Design review of the part built by this model. Coordinates are the model's own, in mm. A direction names the side the tool comes from. Round coordinates to 2 decimals unless told otherwise and drop trailing zeros. Order: outer loops, then holes, each group sorted by start corner. A loop starts at its lowest first (then second) coordinate and runs counter-clockwise, first axis right, second up.
from build123d import *

# Parameters (mm, degrees)
SKETCH3_R           = 4
BOSS_EXTRUDE1_DEPTH = 5.5


with BuildPart() as part:
    # Sketch3 → Boss-Extrude1 (new body)
    with BuildSketch(Plane.XY):
        with BuildLine():
            Line((35.572698846, 9), (-28.927301154, 9))
            Line((-28.927301154, 9), (-32.927301154, 1))
            Line((-32.927301154, 1), (-12.087578676, 2.254578437))
            ThreePointArc((-12.087578676, 2.254578437), (-10.138135968, 1.682819545), (-9, 0))
            ThreePointArc((-9, 0), (0.50116839, -8.986035291), (8.944184499, 1.000781519))
            Line((8.944184499, 1.000781519), (35.848085015, 6.02549586))
            ThreePointArc((35.848085015, 6.02549586), (37.066311281, 7.638281941), (35.572698846, 9))
        make_face()
        Circle(SKETCH3_R, mode=Mode.SUBTRACT)
    extrude(amount=BOSS_EXTRUDE1_DEPTH)


solid = part.part
1) Take a section at A-A on x = 0. Give the boundary of the cut face in (y, z).
Results:
outline: (-9, 0) - (-4, 0) - (-4, 5.5) - (-9, 5.5) - close; (4, 0) - (9, 0) - (9, 5.5) - (4, 5.5) - close
2) Take a section at C-C on z = 3.65. Give the boundary of the cut face in (x, y).
Results:
outline: (-32.93, 1) - (-12.09, 2.25) arc R3 cw to (-9, 0) arc R9 ccw (long way) to (8.94, 1) - (35.85, 6.03) arc R1.5 ccw to (35.57, 9) - (-28.93, 9) - close; hole circle Ø8 at (0, 0)
3) Take a section at B-B on y = -3.25. Give the boundary of the cut face in (x, z), plus the area to 3 significant figures.
Results:
outline: (-8.39, 0) - (-2.33, 0) - (-2.33, 5.5) - (-8.39, 5.5) - close; (2.33, 0) - (8.39, 0) - (8.39, 5.5) - (2.33, 5.5) - close
area: 66.7 mm2
4) For faces 4 (the face through (-22.65, 1.62, 2.71)), 5 (the face through (4, 9, 3)), list the 3-axis set-ups (+Z, -Z, +X, -X, +Y, -Y) from which the entire face can be reached by the end or side of a thin tool; tool diameter is ignored.
Results:
face 4: +Z, -Z, -Y
face 5: +Z, -Z, +X, -X, +Y
5) Clearance check with flat-ended pins moving along their axes: P1, Ø2, axis at y = -4, z = 2.5, coming from the -X side; P2, Ø1.5, axis at y = -2.5, z = 1.5, coming from the +X side; P3, Ø1.5, axis at y = 0.5, z = 2.5, coming from the -X side. State where each tip first meets the part, or that it passes through.
Results:
P1: stops at x = -8.49
P2: stops at x = 8.83
P3: stops at x = -32.93
6) The part is to be moulded in two halves that separate along X. For faces 1 (the face through (-10.16, 1.7, 2.71)), 2 (the face through (37.07, 7.61, 2.71)), 3 (the face through (2, 4, 5.5)), say which applies: released by +X, released by -X, zero draft, split by the parting line, or undercut.
Results:
face 1: undercut
face 2: released by +X
face 3: zero draft
7) To check wall thickness, follow line 1 along Y through (x, z) = (0, 1.85); line 2 along Y through (x, z) = (33, 0.8); line 3 along X through (y, z) = (-3, 4.45). State the ranges of each line that lie inside material, in increasing order.
Results:
line 1: y = -9 to -4, 4 to 9
line 2: y = 5.49 to 9
line 3: x = -8.49 to -2.65, 2.65 to 8.49
8) Take a section at D-D on x = 13. Give the boundary of the cut face in (y, z), plus the area to 3 significant figures.
Results:
outline: (1.76, 0) - (9, 0) - (9, 5.5) - (1.76, 5.5) - close
area: 39.8 mm2
